The listing builds one solid part. Answer for the finished solid, in the listing's coordinates (mm). A direction names the side the tool comes from. Coordinates: 2 decimals unless noted, no trailing zeros. Order: outer loops, then holes, each group sorted by start corner. A loop starts at its lowest first (then second) coordinate and runs counter-clockwise, first axis right, second up. Notation, with made-up numbers: M 52,29.5 L 75,29.5 A25 ccw 75,49.5 Z; hole C 85,2 d7. An arc over 180 degrees is marked long. One line per item, written item: value. Start each with the question number.
Q1. Each of these flat-tipped pins is pushed along its axis until it touches: pin 1 Ø1 at (y, z) = (3, 36.5) entering from +X; pin 2 Ø3 at (y, z) = (5.5, 30) entering from -X; pin 3 Ø1 at (x, y) = (-8, 2) entering from +Z. Where does it stop, or does it pass through?
Q2. The part is cut by section D-D on z = 67. Give the vertices of the cut face in (x, y).
Q3. Determine the mould class of faces 1 (the cylindrical face through (-60.05, 3.13, 63.75)), 2 (the flat face through (-25, 0, 45)), 3 (the cylindrical face through (-11.82, 3.13, 12.79)) for opening direction Z: pulls with the +Z half, pulls with the -Z half, needs draft (parallel to the pull), parting line crosses it, or undercut.
Q4. For faces 4 (the flat face through (-38.79, 3.13, 55.24)), 5 (the cylindrical face through (1, 3, 20)), determine the directions among +Z, -Z, +X, -X, +Y, -Y from which every point of the face is accessible in a straight line to the end or side of a thin tool.
Q5. The part is cut by section C-C on y = 3. Give the vertices of the cut face in (x, z).
Q6. Straight lines are drawn through the part: line 1 along Z through (x, y) = (-39, 2); line 2 along Z through (x, y) = (-51.5, 0.5); line 3 along X through (y, z) = (0.5, 58). For each, find the intervals that lie inside material, in ascending order. Write a range as [from, to].
Q7. The part is cut by section A-A on z = 18.5. Give the vertices of the cut face in (x, y), then the cut area to 3 significant figures.
Q8. The part is cut by section B-B on x = -27. Give the vertices of the cut face in (y, z), then the cut area to 3 significant figures.
```python
from build123d import *

# Parameters (mm, degrees)
BOSS_EXTRUDE1_DEPTH = 6.35


with BuildPart() as part:
    # Sketch1 → Boss-Extrude1 (new body)
    with BuildSketch(Plane(origin=(0, 0, 0), x_dir=(1, 0, 0), z_dir=(0, 1, 0))):
        with BuildLine():
            Line((-12.660316566, -13.672486937), (-14.793671701, -33.72155142))
            ThreePointArc((-14.793671701, -33.72155142), (-15.910435011, -36.619656083), (-18.326632738, -38.571106689))
            Line((-18.326632738, -38.571106689), (-73.332068985, -62.976257477))
            ThreePointArc((-73.332068985, -62.976257477), (-74.387185899, -64.085254343), (-74.349087019, -65.615513872))
            Line((-74.349087019, -65.615513872), (-71.53446378, -71.959239443))
            ThreePointArc((-71.53446378, -71.959239443), (-70.425466914, -73.014356356), (-68.895207385, -72.976257477))
            Line((-68.895207385, -72.976257477), (0.303992163, -42.273530354))
            ThreePointArc((0.303992163, -42.273530354), (2.320082288, -40.814341122), (3.57063844, -38.662606492))
            Line((3.57063844, -38.662606492), (12.082791936, -12.764755482))
            ThreePointArc((12.082791936, -12.764755482), (11.691090758, -12.25206691), (11.120053366, -12.552392867))
            ThreePointArc((11.120053366, -12.552392867), (0.429889276, -20.034212045), (-10.768550895, -13.337036209))
            ThreePointArc((-10.768550895, -13.337036209), (-11.84052795, -12.793656499), (-12.660316566, -13.672486937))
        make_face()
        with BuildLine():
            Line((-59.558046082, -62.405054335), (-20.220801555, -44.680449865))
            ThreePointArc((-20.220801555, -44.680449865), (-18.898273358, -45.181368191), (-19.399191684, -46.503896387))
            Line((-19.399191684, -46.503896387), (-58.736436211, -64.228500857))
            ThreePointArc((-58.736436211, -64.228500857), (-60.058964408, -63.727582531), (-59.558046082, -62.405054335))
        make_face(mode=Mode.SUBTRACT)
    extrude(amount=BOSS_EXTRUDE1_DEPTH)


solid = part.part
```
Output:
1. pin 1: stops at x = 4.45
1. pin 2: stops at x = -14.56
1. pin 3: stops at z = 46.18
2. outline: M -73.73,0 L -55.43,0 L -55.43,6.35 L -73.73,6.35 Z
3. face 1: undercut
3. face 2: needs draft
3. face 3: pulls with the -Z half
4. face 4: +Y, -Y
4. face 5: -Z, +Y, -Y
5. outline: M -74.35,65.62 A2 ccw -73.33,62.98 L -18.33,38.57 A6 cw -14.79,33.72 L -12.66,13.67 A1 ccw -10.77,13.34 A12 cw 11.12,12.55 A0.5 ccw 12.08,12.76 L 3.57,38.66 A6 ccw 0.3,42.27 L -68.9,72.98 A2 ccw -71.53,71.96 Z; hole M -59.56,62.41 L -20.22,44.68 A1 ccw -19.4,46.5 L -58.74,64.23 A1 ccw Z
6. line 1: z = [47.74, 53.14], [55.34, 59.71]
6. line 2: z = [53.29, 58.77], [60.97, 65.26]
6. line 3: x = [-62.12, -49.78], [-44.91, -35.14]
7. outline: M -13.17,0 L -5.88,0 L -5.88,6.35 L -13.17,6.35 Z; M 5.88,0 L 10.2,0 L 10.2,6.35 L 5.88,6.35 Z
7. area: 73.7 mm^2
8. outline: M 0,42.42 L 6.35,42.42 L 6.35,47.74 L 0,47.74 Z; M 0,49.93 L 6.35,49.93 L 6.35,54.39 L 0,54.39 Z
8. area: 62.1 mm^2
